Work out the finished part from the listing and answer in its coordinate system (mm). A direction names the side the tool comes from. Coordinates: 2 decimals unless noted, no trailing zeros. Order: outer loops, then holes, each group sorted by start corner. A loop starts at its lowest first (then second) coordinate and runs counter-clockwise, first axis right, second up. Notation, with made-up numbers: (42, -3.5) - (71, -3.5) arc R18 cw to (71, 18.5) - close; hole circle Ø7 at (37.5, 82). An arc over 180 degrees is marked (long way). Answer as a JSON object with one key per item and string values. Group by question number.
1) Section C-C (x = 7.5) is taken. Give the vertices of the cut face in (y, z).
2) Section A-A (z = 0) is taken. Give the vertices of the cut face in (x, y), plus the area to 3 significant figures.
3) Section B-B (y = -61) is taken. Give the vertices of the cut face in (x, z) (1 decimal), plus the area to 3 significant figures.
4) The mould has two halves that part along X. Classify faces 1 (the face through (23.846, -19.72, -7.509)), 2 (the face through (19.16, -54.79, 2.52)), 3 (the face through (-12, -70, 0)): released by +X, released by -X, zero draft, split by the parting line, or undercut.
5) Each of these flat-tipped pins is pushed along its axis until it touches: P1, Ø8, axis at x = -16.5, z = 3.5, coming from the +Y side; P2, Ø5, axis at y = -28.5, z = 20, coming from the +X side; P3, Ø12, axis at x = -2.5, y = -50.5, coming from the -Z side. Where does it stop, or does it pass through?
6) Section D-D (x = -20) is taken. Give the vertices of the cut face in (y, z), plus the area to 3 significant figures.
7) Find the intervals of material crossed by line 1 along X through (y, z) = (12.5, -15); line 2 along Y through (x, z) = (-14, -16); line 3 along X through (y, z) = (-4, -19), in increasing order.
8) A tool of negligible diameter and unlimited length cuts with its end or side. For faces 4 (the face through (13, -70, 0)), 5 (the face through (0, -40, 0)), from which of +Z, -Z, +X, -X, +Y, -Y can it reach the whole face along a straight path? Write none if from no direction.
Autodesk Inventor part; units mm, degrees
ref_plane "YZ Plane" through (0, 0, 0) normal (1, 0, 0) x (0, 1, 0)
ref_plane "XZ Plane" through (0, 0, 0) normal (0, 1, 0) x (-1, 0, 0)
ref_plane "XY Plane" through (0, 0, 0) normal (0, 0, 1) x (1, 0, 0)
sketch "Sketch1" plane through (0, 0, 0) normal (0, 1, 0) x (-1, 0, 0)
  arc A0 (0, 25) -> (0, -25) centre (0, 0) ccw
  line L0 (0, 25) -> (0, -25)
  dimension "d0" = 50
revolve "Revolution1" add sketch "Sketch1" angle 180 about axis through (0, 0, 25) along (0, 0, 1)
sketch "Sketch2" plane through (0, 0, 0) normal (0, -1, 0) x (1, 0, 0)
  circle A0 centre (0, 0) radius 25
extrude "Extrusion1" add sketch "Sketch2" along normal blind 40
sketch "Sketch3" plane through (0, -40, 0) normal (0, -1, 0) x (1, 0, 0)
  circle A0 centre (-11.7165, 0) radius 6.5669
  circle A1 centre (13.095, 0) radius 6.5681
  point P0 (0, 0)
extrude "Extrusion2" add sketch "Sketch3" along normal blind 30
properties part number "red led now"
Report:
{
 "1": {"outline": "(-70, -3.44) - (-40, -3.44) - (-40, -23.85) - (0, -23.85) arc R23.85 ccw to (0, 23.85) - (-40, 23.85) - (-40, 3.44) - (-70, 3.44) - close"},
 "2": {"outline": "(-25, -40) - (-18.28, -40) - (-18.28, -70) - (-5.15, -70) - (-5.15, -40) - (6.53, -40) - (6.53, -70) - (19.66, -70) - (19.66, -40) - (25, -40) - (25, 0) arc R25 ccw to (-25, 0) - close", "area": "3,770 mm²"},
 "3": {"outline": "circle Ø13.1 at (-11.7, 0); circle Ø13.1 at (13.1, 0)", "area": "271 mm²"},
 "4": {"face 1": "split by the parting line", "face 2": "undercut", "face 3": "zero draft"},
 "5": {"P1": "stops at y = 21.43", "P2": "stops at x = 17.85", "P3": "stops at z = -5.73"},
 "6": {"outline": "(-40, -15) - (0, -15) arc R15 ccw to (0, 15) - (-40, 15) - close", "area": "1,550 mm²"},
 "7": {"line 1": "x = -15.61 to 15.61", "line 2": "y = -40 to 13.15", "line 3": "x = -16.25 to 16.25"},
 "8": {"face 4": "+Z, -Z, +X, -X, -Y", "face 5": "-Y"}
}
